```python
from build123d import *

# Parameters (mm, degrees)
F0_W      = 288.925
F0_H      = 190.5
F1_DEPTH  = 3.175
F3_DEPTH  = 3.175
F5_DEPTH  = 3.175
F6_W      = 288.925
F6_H      = 254
F7_DEPTH  = 3.175
F8_W      = 158.75
F8_H      = 158.75
F9_DEPTH  = 3.175
F12_DEPTH = 69.85
F13_W     = 3.1750007891
F13_H     = 253.9999979416
F13_W_2   = 3.1750009115
F13_H_2   = 253.9999979885
F14_DEPTH = 69.85
F16_DEPTH = 3.175


# Not quite as in the source:
# - ends of sketch curves that miss each other by under 0.0002 mm in the source are joined


with BuildPart() as f1:
    # F0 (on Top) → F1 (new body)
    with BuildSketch(Plane.XY):
        Rectangle(F0_W, F0_H)
    extrude(amount=F1_DEPTH)

    # F2 (on face) → F3 (join)
    with BuildSketch(Plane.XY.offset(3.175)):
        Polygon((-144.4625, -95.25), (-144.4625, 95.25), (-217.4875, 95.25), align=None)
    extrude(amount=-F3_DEPTH)

    # F4 (on face) → F5 (join)
    with BuildSketch(Plane(origin=(0, 0, 0), x_dir=(1, 0, 0), z_dir=(0, 0, -1))):
        Polygon((217.4875, -95.25), (144.4625, 95.25), (144.4625, -95.25), align=None)
    extrude(amount=-F5_DEPTH)

    # F6 (on face) → F7 (join)
    with BuildSketch(Plane.XY.offset(3.175)):
        with Locations((0, -222.25)):
            Rectangle(F6_W, F6_H)
    extrude(amount=-F7_DEPTH)

    # F8 (on face) → F9 (cut)
    with BuildSketch(Plane.XY.offset(3.175)):
        with Locations((0, -211.1248)):
            Rectangle(F8_W, F8_H)
    extrude(amount=-F9_DEPTH, mode=Mode.SUBTRACT)

    # F10 (on face) + F11 (on face) → F12 (join)
    with BuildSketch(Plane.XY.offset(3.175)):
        Polygon((-214.3125, 95.25), (-217.4875, 95.25), (-144.4624992109, -95.2500020584), (-141.2874992109, -95.2500020584), align=None)
    with BuildSketch(Plane.XY.offset(3.175)):
        Polygon((144.4624990885, -95.2500020115), (217.4875, 95.25), (214.3125, 95.25), (141.2874990885, -95.2500020115), align=None)
    extrude(amount=F12_DEPTH)

    # F13 (on face) → F14 (join)
    with BuildSketch(Plane.XY.offset(3.175)):
        with Locations((-142.8749996055, -222.2500010292)):
            Rectangle(F13_W, F13_H)
        with Locations((142.8749995443, -222.2500010058)):
            Rectangle(F13_W_2, F13_H_2)
    extrude(amount=F14_DEPTH)

    # F15 (on face) → F16 (join)
    with BuildSketch(Plane.XY.offset(73.025)):
        Polygon((-153.5540740075, -71.5328504152), (-144.4625, -95.25), (-141.2874992109, -95.2500000226), (-150.3790740075, -71.5328504152), align=None)
        Polygon((-150.3790740075, -71.5328504152), (-141.2874992109, -95.2500020584), (144.4625, -95.2500020584), (153.5540740075, -71.5328504152), align=None)
    extrude(amount=F16_DEPTH)


solid = f1.part
```
Verification items for the finished model (mm, model axes). A direction names the side the tool comes from. Coordinates: 2 decimals unless noted, no trailing zeros. Write each loop counter-clockwise with the first axis right and the second up, starting at its lowest first coordinate (ties: lowest second). Pieces come first, ordered by that corner, then holes. Notation, with made-up numbers: M 11,54 L 62,54 A24 cw 62,87 Z; hole C 31.5,15.25 d1. An arc over 180 degrees is marked long. One line per item, written item: value.
Item 1: Mould release check, pull along X, two halves, no side actions. Record for faces 1 (the flat face through (-1, -349.25, 1)), 2 (the flat face through (-141.287, -224, 38)), 3 (the flat face through (144.462, -224, 37)): pulls with the +X half, pulls with the -X half, needs draft (parallel to the pull), parting line crosses it, or undercut.
Check sheet entries:
face 1: needs draft
face 2: undercut
face 3: pulls with the +X half
Item 2: Section check C-C, the plane x = 29. Record the boundary of the cut face in (y, z) (3 decimals), plus the area to 3 significant figures.
Check sheet entries:
outline: M -349.25,0 L -290.5,0 L -290.5,3.175 L -349.25,3.175 Z; M -131.75,0 L 95.25,0 L 95.25,3.175 L -131.75,3.175 Z; M -95.25,73.025 L -71.533,73.025 L -71.533,76.2 L -95.25,76.2 Z
area: 983 mm^2
Item 3: Gauge pin test, flat ends, axial feed: pin 1 Ø1.5 at (y, z) = (-77, 59) entering from +X; pin 2 Ø1 at (x, y) = (-142.5, -167.5) entering from +Z (3 decimals); pin 3 Ø2.5 at (x, z) = (63.5, 75) entering from +Y; pin 4 Ø20 at (x, y) = (-196, -7.5) entering from +Z. Record the tip position at first contact, or that the pin passes through.
Check sheet entries:
pin 1: stops at x = 151.75
pin 2: stops at z = 73.025
pin 3: stops at y = -71.53
pin 4: passes through
Item 4: Section check A-A, the plane y = -170. Record the boundary of the cut face in (x, z) (1 decimal).
Check sheet entries:
outline: M -144.5,0 L -79.4,0 L -79.4,3.2 L -141.3,3.2 L -141.3,73 L -144.5,73 Z; M 79.4,0 L 144.5,0 L 144.5,73 L 141.3,73 L 141.3,3.2 L 79.4,3.2 Z
Item 5: Section check D-D, the plane x = 130.5. Record the boundary of the cut face in (y, z) (3 decimals).
Check sheet entries:
outline: M -349.25,0 L 95.25,0 L 95.25,3.175 L -349.25,3.175 Z; M -95.25,73.025 L -71.533,73.025 L -71.533,76.2 L -95.25,76.2 Z
Item 6: Access from +Z, -Z, +X, -X, +Y, -Y to the whole of each face (thin tool, end or side, straight path). Record for faces 4 (the flat face through (-144.463, -224, 36)), 5 (the flat face through (141.287, -224, 38)), 6 (the flat face through (-2, -83, 76.2)).
Check sheet entries:
face 4: +Z, -Z, -X, -Y
face 5: +Z, +Y, -Y
face 6: +Z, +X, -X, +Y, -Y
Item 7: Scan lines: line 1 along X through (y, z) = (-284, 61); line 2 along Z through (x, y) = (-77.5, -59.5) (3 decimals); line 3 along Z through (x, y) = (-131, -93) (3 decimals). Record each from-to range of solid material in increasing order.
Check sheet entries:
line 1: x = -144.46 to -141.29, 141.29 to 144.46
line 2: z = 0 to 3.175
line 3: z = 0 to 3.175, 73.025 to 76.2
